Build history of the part. All positions in model axes, mm. A direction names the side the tool comes from. Give positions to 0.01 mm unless a question says otherwise; leave off trailing zeros. Order: outer loops, then holes, each group sorted by start corner. A loop starts at its lowest first (then second) coordinate and runs counter-clockwise, first axis right, second up. Notation, with made-up numbers: M -28,-2 L 19,-2 A12 cw 19,8 Z; hole C 2,48.25 d7. An arc over 180 degrees is marked long. Use CSV: the item, a comma, the result in double quotes. Start each with the question number.
Item 1: Band-saw the part on D-D on y = 8. Write the cut outline in (x, z).
Item 2: Pin check, flat tips, straight feed: P1, Ø3.5, axis at y = -13.21, z = 7.5, coming from the +X side; P2, Ø3, axis at y = -4.5, z = 7.5, coming from the +X side. Stop position of each tip, or through.
Item 3: Band-saw the part on C-C on z = 10.5. Write the cut outline in (x, y), plus the area to 3 significant figures.
Item 4: Two-plate mould, pull along Z, no slides. Class faces 1 (the cylindrical face through (3.605, -16.639, 14.399)), 2 (the flat face through (-0.832, -3, 7)), 3 (the cylindrical face through (3.73, -11.696, 7.164)), 4 (the cylindrical face through (3.73, 5.255, 7.298)): pulls with the +Z half, pulls with the -Z half, needs draft (parallel to the pull), parting line crosses it, or undercut.
Item 5: Band-saw the part on B-B on x = 4.5. Write the cut outline in (y, z).
Item 6: Band-saw the part on A-A on z = 7.5. Write the cut outline in (x, y), plus the area to 3 significant figures.
Item 7: Which spindle directions (+Z, -Z, +X, -X, +Y, -Y) get a long thin tool onto all of the face, cutting with end or side? Do faces 5 (the flat face through (4, -17.209, 7)), 6 (the flat face through (3.168, -3, 7)). Say none if no direction does.
Item 8: Wall check: line 1 along Y through (x, z) = (3, 7.5); line 2 along Y through (x, z) = (1.5, 8.75); line 3 along Y through (x, z) = (5.25, 6.25). Give the ranges that are in metal, low to high.
Autodesk Inventor part; units mm, degrees
ref_plane "YZ Plane" through (0, 0, 0) normal (1, 0, 0) x (0, 1, 0)
ref_plane "XZ Plane" through (0, 0, 0) normal (0, 1, 0) x (-1, 0, 0)
ref_plane "XY Plane" through (0, 0, 0) normal (0, 0, 1) x (1, 0, 0)
sketch "Sketch2" plane through (0, 0, 0) normal (0, 0, 1) x (1, 0, 0)
  line L0 (3.1675, -3.2086) -> (3.1675, 0.0414)
  arc A0 (8.1675, 2.7916) -> (3.1675, 0.0414) centre (8.1675, -3.1285) ccw
  line L1 (5.3308, -15.8516) -> (5.3308, -15.8516)
  line L2 (8.1675, 2.7916) -> (8.1675, 10.7916)
  line L3 (3.1675, -3.2086) -> (3.1675, -6.4586)
  arc A1 (3.1675, -6.4586) -> (8.1675, -9.2089) centre (8.1675, -3.2888) ccw
  line L4 (8.1675, -9.2089) -> (8.1675, -17.2089)
  line L5 (8.1675, 10.7916) -> (-0.8325, 10.7916)
  line L6 (8.1675, -17.2089) -> (-0.8325, -17.2089)
  line L7 (-0.8325, 10.7916) -> (-0.8325, -17.2089)
  point P0 (0, 0)
  point P1 (8.1675, -9.2089)
  dimension "d10" = 9
  dimension "d11" = 4
extrude "Extrusion2" add sketch "Sketch2" along normal blind 15
ref_plane "Work Plane1" through (-0.8325, -3.2086, 0) normal (0, 1, 0) x (1, 0, 0)
sketch "Sketch3" plane through (-0.8325, -17.2089, 0) normal (-1, 0, 0) x (0, 0, 1)
  line L0 (0, 28.0006) -> (0, 0)
  line L1 (0, 0) -> (15, 0)
  line L2 (0, 28.0006) -> (15, 28.0006)
  point P0 (7.5, 4)
  point P1 (7.5, 24.0006)
  point P2 (7.5, 0)
  point P3 (7.5, 28.0006)
  dimension "d16" = 7.5
  dimension "d17" = 4
  dimension "d18" = 4
  dimension "d19" = 7.5
hole "Hole1" at (-0.8325, -13.2089, 7.5) at (-0.8325, 6.7916, 7.5) direction (1, 0, 0) diameter 3.1 end through all
fillet "Fillet1" radius 2 4 edges at (3.6675, 10.7916, 15) (3.6675, 10.7916, 0) (3.6675, -17.2089, 0) (3.6675, -17.2089, 15)
properties part number "podstawka silnika_CPY" material "ABS Plastic"
Model answer:
1,outline,"M -0.83,0 L 8.17,0 L 8.17,6.53 L -0.83,6.53 Z; M -0.83,8.47 L 8.17,8.47 L 8.17,15 L -0.83,15 Z"
2,P1,"stops at x = 8.17"
2,P2,"stops at x = 3.17"
3,outline,"M -0.83,-17.21 L 8.17,-17.21 L 8.17,-9.21 A5.92 cw 3.17,-6.46 L 3.17,0.04 A5.92 cw 8.17,2.79 L 8.17,10.79 L -0.83,10.79 Z"
3,area,"200 mm^2"
4,face 1,"pulls with the +Z half"
4,face 2,"needs draft"
4,face 3,"undercut"
4,face 4,"undercut"
5,outline,"M -17.21,2 A2 ccw -15.21,0 L -7.94,0 L -7.94,15 L -15.21,15 A2 ccw -17.21,13 Z; M 1.52,0 L 8.79,0 A2 ccw 10.79,2 L 10.79,13 A2 ccw 8.79,15 L 1.52,15 Z; hole C -13.21,7.5 d3.1; hole C 6.79,7.5 d3.1"
6,outline,"M -0.83,-17.21 L 8.17,-17.21 L 8.17,-14.76 L -0.83,-14.76 Z; M -0.83,-11.66 L 8.17,-11.66 L 8.17,-9.21 A5.92 cw 3.17,-6.46 L 3.17,0.04 A5.92 cw 8.17,2.79 L 8.17,5.24 L -0.83,5.24 Z; M -0.83,8.34 L 8.17,8.34 L 8.17,10.79 L -0.83,10.79 Z"
6,area,"144 mm^2"
7,face 5,"+Z, -Z, +X, -X, -Y"
7,face 6,"+Z, -Z, +X"
8,line 1,"y = -17.21 to -14.76, -11.66 to 5.24, 8.34 to 10.79"
8,line 2,"y = -17.21 to -14.13, -12.29 to 5.88, 7.71 to 10.79"
8,line 3,"y = -17.21 to -14.13, -12.29 to -8.44, 2.02 to 5.88, 7.71 to 10.79"
